from build123d import *

# Parameters (mm, degrees)
MODEL_R             = 0.925
MODEL_R_2           = 0.875
BOSS_EXTRUDE1_DEPTH = 3
FILLET2_R           = 0.5
FILLET3_R           = 1


with BuildPart() as part:
    # Model → Boss-Extrude1 (new body)
    with BuildSketch(Plane.XY):
        Polygon((142.344747242, 270.871489374), (153.37187249, 271.263447748), (162.091473536, 274.767362889), (160.85900272, 279.367807803), (179.260689602, 284.297666211), (178.028627015, 288.898354165), (208.019481767, 296.93522173), (209.252454514, 292.334187025), (227.65276755, 297.263677376), (230.276304619, 287.470798216), (275.446186014, 299.571346393), (298.39980436, 213.909597233), (260.87259576, 203.855963236), (255.943287021, 222.255598366), (248.650938057, 220.301667543), (251.115775513, 211.101166572), (220.422247557, 202.878292884), (219.189771603, 207.477473721), (213.081966369, 205.841177268), (214.314693354, 201.241059665), (196.039346948, 196.343682115), (196.007810089, 177.840578221), (186.702312667, 152.27893851), (161.565977706, 161.426447529), (132.435827139, 161.934428279), (107.399642776, 152.824765622), (97.980730454, 178.710864183), (99.858189105, 195.997881416), (81.758593313, 200.846808858), (82.991121062, 205.447466285), (76.882860045, 207.083884844), (75.650856625, 202.485184579), (44.956891994, 210.708175253), (47.421773629, 219.90863481), (40.129543563, 221.862285479), (35.199939127, 203.463086712), (-2.32684459, 213.517448416), (20.785545351, 299.774827661), (65.955825932, 287.671594898), (68.42160019, 296.872525865), (86.820985153, 291.940533454), (88.054439652, 296.542595671), (118.044472643, 288.503706576), (116.812112756, 283.905728394), (135.211333861, 278.973779905), (133.979081507, 274.376202933), align=None)
        with Locations((23.035554, 295.877718337)):
            Circle(MODEL_R, mode=Mode.SUBTRACT)
        with Locations((109.301822433, 156.902965293)):
            Circle(MODEL_R, mode=Mode.SUBTRACT)
        with Locations((184.800560745, 156.35733766)):
            Circle(MODEL_R, mode=Mode.SUBTRACT)
        with Locations((193.847437398, 289.84318413)):
            Circle(MODEL_R, mode=Mode.SUBTRACT)
        with Locations((102.225689846, 289.449650012)):
            Circle(MODEL_R, mode=Mode.SUBTRACT)
        with Locations((273.19609114, 295.674286852)):
            Circle(MODEL_R_2, mode=Mode.SUBTRACT)
        with Locations((1.570241786, 215.767496811)):
            Circle(MODEL_R, mode=Mode.SUBTRACT)
        with Locations((294.502731407, 216.159668876)):
            Circle(MODEL_R_2, mode=Mode.SUBTRACT)
        with Locations((80.760413887, 209.339268578)):
            Circle(MODEL_R, mode=Mode.SUBTRACT)
        with Locations((215.312231294, 209.732861073)):
            Circle(MODEL_R, mode=Mode.SUBTRACT)
        with Locations((133.281102646, 207.339464548)):
            Circle(MODEL_R, mode=Mode.SUBTRACT)
        with Locations((162.46850521, 207.598897954)):
            Circle(MODEL_R, mode=Mode.SUBTRACT)
        with Locations((142.522359716, 244.531276159)):
            Circle(MODEL_R, mode=Mode.SUBTRACT)
        with Locations((153.549484965, 244.723703681)):
            Circle(MODEL_R, mode=Mode.SUBTRACT)
        Polygon((241.30271159, 224.544411578), (243.767491017, 215.34412721), (224.664804007, 210.226469096), (223.432328054, 214.825649934), (205.733277658, 210.084029615), (206.966112962, 205.483507804), (188.744476932, 200.600523414), (190.038361872, 195.770837942), (170.765567452, 190.607607624), (150.690394167, 265.500431998), (169.439649748, 270.524806438), (168.207287216, 275.124847165), (186.60841776, 280.054556529), (185.376246939, 284.655648642), (203.777033628, 289.586641337), (205.009898064, 284.986010813), (223.409806911, 289.915392881), (226.033325469, 280.122582817), (271.203498451, 292.223209107), (272.169435546, 292.481986095), (292.017165355, 218.411256738), (291.05122826, 218.15247975), (265.115556398, 211.204247731), (264.149619304, 210.945470743), (259.219574531, 229.345102127), align=None, mode=Mode.SUBTRACT)
        Polygon((91.063082461, 284.591613875), (72.663861356, 289.523562363), (70.198239559, 280.323200295), (25.028202346, 292.426367848), (24.062275945, 292.68518475), (4.05571522, 218.019020829), (5.0216469, 217.76022363), (30.957132238, 210.811459981), (31.923058639, 210.55264308), (36.852366702, 228.951863077), (54.770081908, 224.151554257), (52.305208977, 214.951127188), (71.407895987, 209.833469074), (72.639899407, 214.432169339), (90.339405557, 209.690426923), (89.106877808, 205.089769496), (107.149713912, 200.256048118), (105.814746135, 195.273012707), (125.26498777, 190.062243831), (145.381260936, 265.108396206), (126.630323598, 270.134062294), (127.862619282, 274.731800932), (109.463398178, 279.663749421), (110.695758065, 284.261727603), (92.29653696, 289.193676092), align=None, mode=Mode.SUBTRACT)
        Polygon((104.096364698, 179.45072575), (110.986427135, 160.514692668), (131.428930231, 167.95289908), (146.304188304, 173.365408471), (162.674398087, 167.40803076), (183.116533861, 159.968814913), (190.009613349, 178.903688177), (153.172596304, 192.31106529), (147.151959777, 175.767027333), (140.930891121, 192.858221652), align=None, mode=Mode.SUBTRACT)
    extrude(amount=-BOSS_EXTRUDE1_DEPTH)

    # Fillet2
    fillet2_edges = [part.edges().sort_by_distance(p)[0] for p in [
        (147.151959777, 175.767027333, -1.5),
    ]]
    fillet(fillet2_edges, radius=FILLET2_R)

    # Fillet3
    fillet3_edges = [part.edges().sort_by_distance(p)[0] for p in [
        (-2.32684459, 213.517448416, -1.5),
        (20.785545351, 299.774827661, -1.5),
        (68.42160019, 296.872525865, -1.5),
        (88.054439652, 296.542595671, -1.5),
        (118.044472643, 288.503706576, -1.5),
        (135.211333861, 278.973779905, -1.5),
        (160.85900272, 279.367807803, -1.5),
        (178.028627015, 288.898354165, -1.5),
        (208.019481767, 296.93522173, -1.5),
        (227.65276755, 297.263677376, -1.5),
        (275.446186014, 299.571346393, -1.5),
        (298.39980436, 213.909597233, -1.5),
        (260.87259576, 203.855963236, -1.5),
        (251.115775513, 211.101166572, -1.5),
        (220.422247557, 202.878292884, -1.5),
        (214.314693354, 201.241059665, -1.5),
        (186.702312667, 152.27893851, -1.5),
        (107.399642776, 152.824765622, -1.5),
        (81.758593313, 200.846808858, -1.5),
        (75.650856625, 202.485184579, -1.5),
        (44.956891994, 210.708175253, -1.5),
        (35.199939127, 203.463086712, -1.5),
    ]]
    fillet(fillet3_edges, radius=FILLET3_R)


solid = part.part
Geometry check sheet. Reference: the model listing, model coordinates, mm. A direction names the side the tool comes from. Round coordinates to 2 decimals unless told otherwise and drop trailing zeros. Order: outer loops, then holes, each group sorted by start corner. A loop starts at its lowest first (then second) coordinate and runs counter-clockwise, first axis right, second up. Notation, with made-up numbers: M 35,63 L 75,63 A31 cw 75,87 Z; hole C 7.5,1.5 d2. An arc over 180 degrees is marked long. Answer in a Markdown table with one row per item.
(1) Sectioned sample at B-B, the plane y = 237.5. Record the cut outline in (x, z).
Responses:
| item | result |
|---|---|
| outline | M 4.1,-3 L 9.28,-3 L 9.28,0 L 4.1,0 Z; M 137.98,-3 L 158.2,-3 L 158.2,0 L 137.98,0 Z; M 286.9,-3 L 292.08,-3 L 292.08,0 L 286.9,0 Z |
(2) Sectioned sample at A-A, the plane y = 256.5. Record the cut outline in (x, z), and give its area (3 significant figures).
Responses:
| item | result |
|---|---|
| outline | M 9.19,-3 L 14.37,-3 L 14.37,0 L 9.19,0 Z; M 143.07,-3 L 153.1,-3 L 153.1,0 L 143.07,0 Z; M 281.81,-3 L 286.99,-3 L 286.99,0 L 281.81,0 Z |
| area | 61.1 mm² |
(3) Draft check along Y on faces 1 (the face through (191.59, 165.7, -1.48)), 2 (the face through (150.436, 184.791, -1.479)), 3 (the face through (135.182, 227.06, -1.479)), 4 (the face through (9.071, 256.056, -1.479)). Enter one of: released by +Y, released by -Y, zero draft, split by the parting line, or undercut.
Responses:
| item | result |
|---|---|
| face 1 | released by -Y |
| face 2 | undercut |
| face 3 | undercut |
| face 4 | released by +Y |
(4) Go/stop test with flat-tipped pins: P1, Ø1.5, axis at y = 200.5, z = -2, coming from the +X side; P2, Ø1.5, axis at y = 259.5, z = -0.5, coming from the +X side; P3, Ø1.5, axis at x = 88, z = -1.5, coming from the +Y side. Record where each tip stops, or that it passes through.
Responses:
| item | result |
|---|---|
| P1 | stops at x = 213.81 |
| P2 | stops at x = 286.38 |
| P3 | stops at y = 296.32 |
(5) Tool access check on faces 5 (the face through (235.97, 207.044, -1.479)), 6 (the face through (16.686, 208.424, -1.479)), 7 (the face through (192.828, 292.864, -1.479)), 8 (the face through (14.199, 255.875, -1.479)). Record the directions out of +Z, -Z, +X, -X, +Y, -Y that give a thin tool (end or side, any length) a straight path to the whole face; none if there is none.
Responses:
| item | result |
|---|---|
| face 5 | +Z, -Z, -Y |
| face 6 | +Z, -Z, -X, -Y |
| face 7 | +Z, -Z, +Y |
| face 8 | +Z, -Z |
(6) Scan lines: probe 1 along X at (y, z) = (255.5, -1.3); probe 2 along X at (y, z) = (232.5, -0.45); probe 3 along X at (y, z) = (245.5, -0.7). Record each from-to range of solid material in increasing order. Write a range as from..to.
Responses:
| item | result |
|---|---|
| probe 1 | x = 8.92..14.1, 142.81..153.37, 282.08..287.26 |
| probe 2 | x = 2.76..7.94, 136.64..159.54, 288.24..293.42 |
| probe 3 | x = 6.24..11.42, 140.13..153.05, 154.05..156.05, 284.76..289.93 |
(7) Sectioned sample at C-C, the plane z = -0.85. State how many separate pieces and enclosed holes the cut face has, and give its area (3 significant figures).
Responses:
| item | result |
|---|---|
| separate pieces | 1 |
| enclosed holes | 17 |
| area | 7,750 mm² |
